```python
from build123d import *

# Parameters (mm, degrees)
EXTRUDE_2_DEPTH     = 34.78
CUT_EXTRUDE_1_REACH = 68.736
SKETCH_2_W          = 20
SKETCH_2_H          = 20
CHAMFER_1_SIZE      = 1
CUT_EXTRUDE_START   = -44.54
SKETCH_3_R          = 2
CUT_EXTRUDE_2_DEPTH = 44.54
SKETCH_4_R          = 2
CUT_EXTRUDE_3_DEPTH = 5
SKETCH_6_W          = 34.54
SKETCH_6_H          = 5
EXTRUDE_3_DEPTH     = 10
SKETCH_8_R          = 2
CUT_EXTRUDE_4_DEPTH = 5
EXTRUDE_START       = -2
EXTRUDE_4_DEPTH     = 5


with BuildPart() as part:
    # 草图1 → 凸台-拉伸2 (new body)
    with BuildSketch(Plane.XY):
        Polygon((0, 0), (0, 35.5), (5, 35.5), (5, 5), (39.54, 5), (39.54, 35.5), (44.54, 35.5), (44.54, 0), align=None)
    extrude(amount=EXTRUDE_2_DEPTH)

    # 切除-拉伸1: up to this face of the body (flat: up to its plane)
    cut_extrude_1_end = Plane(part.part.faces().sort_by_distance((0, 17.75, 17.39))[0])
    # 草图2 → 切除-拉伸1 (cut, up to the picked face)
    with BuildSketch(Plane(origin=(44.54, 0, 0), x_dir=(0, 0, -1), z_dir=(1, 0, 0)), mode=Mode.PRIVATE) as cut_extrude_1_sk1:
        with Locations((-17.28, 15)):
            Rectangle(SKETCH_2_W, SKETCH_2_H)
    cut_extrude_1_tool1 = split(extrude(cut_extrude_1_sk1.sketch, amount=-CUT_EXTRUDE_1_REACH, mode=Mode.PRIVATE), bisect_by=cut_extrude_1_end, keep=Keep.BOTH, mode=Mode.PRIVATE)
    add(cut_extrude_1_tool1.solids().sort_by(Axis((44.54, 15, 17.28), (-1, 0, 0)))[0], mode=Mode.SUBTRACT)

    # 倒角1
    chamfer_1_edges = [part.edges().sort_by_distance(p)[0] for p in [
        (44.54, 17.75, 0),
        (22.27, 0, 0),
        (0, 0, 17.39),
        (44.54, 35.5, 17.39),
        (44.54, 0, 17.39),
        (0, 17.75, 34.78),
        (22.27, 0, 34.78),
        (0, 17.75, 0),
        (44.54, 17.75, 34.78),
    ]]
    chamfer(chamfer_1_edges, length=CHAMFER_1_SIZE)

    # 草图3 → 切除-拉伸2 (cut)
    with BuildSketch(Plane(origin=(44.54, 0, 0), x_dir=(0, 0, -1), z_dir=(1, 0, 0)).offset(CUT_EXTRUDE_START)):
        with Locations((-30.53, 19.5)):
            Circle(SKETCH_3_R)
        with Locations((-4.25, 19.5)):
            Circle(SKETCH_3_R)
        with Locations((-4.25, 29.5)):
            Circle(SKETCH_3_R)
        with BuildLine():
            ThreePointArc((-31.619976701, 31.176887233), (-32.53, 29.5), (-31.619976701, 27.823112767))
            Line((-31.619976701, 27.823112767), (-30.53, 29.5))
            Line((-30.53, 29.5), (-31.619976701, 31.176887233))
        make_face()
        with BuildLine():
            Line((-30.53, 29.5), (-31.619976701, 27.823112767))
            ThreePointArc((-31.619976701, 27.823112767), (-30.53, 27.5), (-29.440023299, 27.823112767))
            Line((-29.440023299, 27.823112767), (-30.53, 29.5))
        make_face()
        with BuildLine():
            Line((-30.53, 29.5), (-29.440023299, 27.823112767))
            ThreePointArc((-29.440023299, 27.823112767), (-28.772167044, 28.546048587), (-28.53, 29.5))
            ThreePointArc((-28.53, 29.5), (-28.772167044, 30.453951413), (-29.440023299, 31.176887233))
            Line((-29.440023299, 31.176887233), (-30.53, 29.5))
        make_face()
        with BuildLine():
            ThreePointArc((-29.440023299, 31.176887233), (-30.53, 31.5), (-31.619976701, 31.176887233))
            Line((-31.619976701, 31.176887233), (-30.53, 29.5))
            Line((-30.53, 29.5), (-29.440023299, 31.176887233))
        make_face()
    extrude(amount=CUT_EXTRUDE_2_DEPTH, mode=Mode.SUBTRACT)

    # 草图4 → 切除-拉伸3 (cut)
    with BuildSketch(Plane.XZ):
        with Locations(Location((12.27, 7.39, 0), (0, 0, 270))):
            Circle(SKETCH_4_R)
        with Locations(Location((12.27, 27.39, 0), (0, 0, 270))):
            Circle(SKETCH_4_R)
        with Locations(Location((32.27, 27.39, 0), (0, 0, 270))):
            Circle(SKETCH_4_R)
        with Locations(Location((32.27, 7.39, 0), (0, 0, 270))):
            Circle(SKETCH_4_R)
    extrude(amount=-CUT_EXTRUDE_3_DEPTH, mode=Mode.SUBTRACT)

    # 草图6 → 凸台-拉伸3 (add)
    with BuildSketch(Plane(origin=(0, 5, 0), x_dir=(1, 0, 0), z_dir=(0, 1, 0))):
        with Locations((22.27, -2.5)):
            Rectangle(SKETCH_6_W, SKETCH_6_H)
    extrude(amount=EXTRUDE_3_DEPTH)

    # 草图8 → 切除-拉伸4 (cut)
    with BuildSketch(Plane.XY.offset(5)):
        with Locations((12.27, 10)):
            Circle(SKETCH_8_R)
        with Locations((32.27, 10)):
            Circle(SKETCH_8_R)
    extrude(amount=-CUT_EXTRUDE_4_DEPTH, mode=Mode.SUBTRACT)

    # 草图9 → 凸台-拉伸4 (add)
    with BuildSketch(Plane.XY.offset(34.78).offset(EXTRUDE_START)):
        Polygon((44.54, 34.5), (44.54, 1), (44.54, 0), (43.54, 0), (1, 0), (0, 0), (0, 1), (0, 35.5), (1, 35.5), (5, 35.5), (5, 5), (39.54, 5), (39.54, 35.5), (44.54, 35.5), align=None)
    extrude_4 = extrude(amount=EXTRUDE_4_DEPTH)

    # 镜向1: 凸台-拉伸4 across plane
    add(extrude_4.mirror(Plane(origin=(0, 0, 17.39), x_dir=(1, 0, 0), z_dir=(0, 0, -1))))


solid = part.part
```
Check sheet for the modelled part. Datum: model origin and axes. Units: mm. A direction names the side the tool comes from. Round coordinates to 2 decimals unless told otherwise and drop trailing zeros. Order: outer loops, then holes, each group sorted by start corner. A loop starts at its lowest first (then second) coordinate and runs counter-clockwise, first axis right, second up. Notation, with made-up numbers: (31, 70) - (52, 70) arc R18 cw to (52, 87) - close; hole circle Ø11 at (-40, 38.25). An arc over 180 degrees is marked (long way). Answer as CSV lines item,"result". Start each with the question number.
1) Section check C-C (y = 3.5). Record the cut outline in (x, z), then the cut area to 3 significant figures.
2) Draft check along Z on faces 1 (the face through (2.465, 27.548, 4.684)), 2 (the face through (19.1, 4.7, -3)), 3 (the face through (12.01, 11.983, 2.535)), 4 (the face through (22, 5, 21)). Enter one of: +Z half, -Z half, draft (parallel to the pull), parting line (faces both ways), or undercut.
3) Tool access check on faces 5 (the face through (23, 10, 0)), 6 (the face through (19.1, 4.7, 37.78)), 7 (the face through (10.496, 2.465, 26.467)), 8 (the face through (22, 15, 2)), 9 (the face through (42, 15, 27.28)). Record the directions out of +Z, -Z, +X, -X, +Y, -Y that give a thin tool (end or side, any length) a straight path to the whole face; none if there is none.
4) Section check A-A (x = 32.27). Record the cut outline in (y, z), then the cut area to 3 significant figures.
5) Scan lines: probe 1 along X at (y, z) = (3.3, 27.39); probe 2 along Z at (x, y) = (1.75, 19.5); probe 3 along Y at (x, z) = (1.55, 4.25). Record each from-to range of solid material in increasing order.
6) Section check B-B (z = 4.25). Give the number of separate pieces and of enclosed holes in the cut face, then the cut area to 3 significant figures.
7) Depth check by flat-ended pin: pin 1 (6 mm diameter, centred on x = 21, z = 23, fed in from +Y); pin 2 (6 mm diameter, centred on x = 25, z = 9, fed in from -Y); pin 3 (1 mm diameter, centred on x = 21.5, y = 17, fed in from +Z). Enter the tip coordinate at first touch or a pass-through.
Determined:
1,outline,"(0, -3) - (44.54, -3) - (44.54, 37.78) - (0, 37.78) - close; hole circle Ø4 at (12.27, 7.39); hole circle Ø4 at (12.27, 27.39); hole circle Ø4 at (32.27, 7.39); hole circle Ø4 at (32.27, 27.39)"
1,area,"1,770 mm^2"
2,face 1,"undercut"
2,face 2,"-Z half"
2,face 3,"draft"
2,face 4,"undercut"
3,face 5,"-Z, +Y"
3,face 6,"+Z, +X, -X, +Y, -Y"
3,face 7,"+Y, -Y"
3,face 8,"+Z, -Z, +Y"
3,face 9,"+X, -X"
4,outline,"(0, -3) - (5, -3) - (5, 0) - (8, 0) - (8, 5) - (5, 5) - (5, 5.39) - (0, 5.39) - close; (0, 9.39) - (5, 9.39) - (5, 25.39) - (0, 25.39) - close; (0, 29.39) - (5, 29.39) - (5, 37.78) - (0, 37.78) - close; (12, 0) - (15, 0) - (15, 5) - (12, 5) - close"
4,area,"194 mm^2"
5,probe 1,"0 to 10.27, 14.27 to 30.27, 34.27 to 44.54"
5,probe 2,"-3 to 2.25, 6.25 to 7.28, 27.28 to 28.53, 32.53 to 37.78"
5,probe 3,"0 to 17.5, 21.5 to 27.5, 31.5 to 35.5"
6,separate pieces,"5"
6,enclosed holes,"2"
6,area,"766 mm^2"
7,pin 1,"y = 5"
7,pin 2,"y = 0"
7,pin 3,"through"
